Autodesk Inventor part; units mm, degrees
ref_plane "YZ Plane" through (0, 0, 0) normal (1, 0, 0) x (0, 1, 0)
ref_plane "XZ Plane" through (0, 0, 0) normal (0, 1, 0) x (-1, 0, 0)
ref_plane "XY Plane" through (0, 0, 0) normal (0, 0, 1) x (1, 0, 0)
sketch "Sketch1" plane through (0, 0, 0) normal (1, 0, 0) x (0, 1, 0)
  circle A0 centre (0, -12.7) radius 2.0955
  line L0 (0, 6.35) -> (76.2, 6.35)
  circle A1 centre (0, -38.1) radius 2.0955
  line L1 (-59.2019, -57.15) -> (76.2, -57.15)
  line L2 (76.2, 6.35) -> (96.8375, 6.35)
  line L3 (100.0125, 3.175) -> (100.0125, 1.3151)
  line L4 (95.5224, -3.175) -> (76.1708, -3.175)
  line L5 (76.1708, -47.625) -> (95.5224, -47.625)
  line L6 (100.0125, -52.1151) -> (100.0125, -53.975)
  line L7 (96.8375, -57.15) -> (76.2, -57.15)
  line L8 (99.0826, -0.9299) -> (97.7674, -2.2451)
  line L9 (97.7674, -48.5549) -> (99.0826, -49.8701)
  arc A2 (100.0125, 3.175) -> (96.8375, 6.35) centre (96.8375, 3.175) ccw
  arc A3 (99.0826, -0.9299) -> (100.0125, 1.3151) centre (96.8375, 1.3151) ccw
  arc A4 (95.5224, -3.175) -> (97.7674, -2.2451) centre (95.5224, 0) ccw
  arc A5 (97.7674, -48.5549) -> (95.5224, -47.625) centre (95.5224, -50.8) ccw
  arc A6 (100.0125, -52.1151) -> (99.0826, -49.8701) centre (96.8375, -52.1151) ccw
  arc A7 (96.8375, -57.15) -> (100.0125, -53.975) centre (96.8375, -53.975) ccw
  line L10 (59.0099, -3.175) -> (76.1708, -3.175)
  line L11 (76.1708, -47.625) -> (59.0099, -47.625)
  line L12 (0, 6.35) -> (-60.325, 6.35)
  arc A8 (-60.325, 6.35) -> (-59.8788, -6.3343) centre (-60.325, 0) ccw
  arc A9 (-59.8927, -44.5648) -> (-59.2019, -57.15) centre (-60.325, -50.9001) ccw
  line L13 (6.35, -12.7) -> (6.35, -38.1)
  line L14 (-5.5228, -38.1) -> (-5.5228, -12.0308)
  line L15 (-59.8788, -6.3343) -> (-15.0243, -3.175)
  line L16 (15.875, -3.175) -> (59.0099, -3.175)
  line L17 (15.875, -47.625) -> (59.0099, -47.625)
  line L18 (15.875, -3.175) -> (6.35, -12.7)
  line L19 (6.35, -38.1) -> (15.875, -47.625)
  line L20 (-5.5228, -38.1) -> (-15.0478, -47.625)
  line L21 (-15.0243, -3.175) -> (-5.5228, -12.0308)
  line L22 (-15.0478, -47.625) -> (-59.8927, -44.5648)
  circle A10 centre (-50.8, 0) radius 2.0955
  circle A11 centre (-50.8, -50.8) radius 2.0955
  point P0 (5.4993, -3.175)
  point P1 (0, -57.15)
  point P2 (5.4993, -47.625)
  point P3 (100.0125, -3.175)
  point P4 (100.0125, -47.625)
  point P5 (100.0125, -57.15)
  point P6 (100.0125, 0)
  point P7 (96.8375, -3.175)
  point P8 (96.8375, -47.625)
  point P9 (100.0125, -50.8)
  point P10 (38.1, 6.35)
  point P11 (-5.5228, -2.5058)
  point P12 (-5.5228, -47.625)
  point P13 (85.8466, -3.175)
  point P14 (6.35, -3.175)
  point P15 (6.35, -47.625)
  point P16 (0, 0)
  dimension "d0" = 4.191
  dimension "d6" = 4.191
  dimension "d15" = 3.175
  dimension "d16" = 3.175
  dimension "d17" = 3.175
  dimension "d18" = 3.175
  dimension "d19" = 3.175
  dimension "d29" = 9.525
  dimension "d30" = 9.525
  dimension "d31" = 9.525
  dimension "d32" = 9.525
  dimension "d34" = 9.525
  dimension "d35" = 9.525
  dimension "d36" = 9.525
  dimension "d37" = 9.525
  dimension "d38" = 9.525
  dimension "d39" = 12.7
  dimension "d40" = 12.7
  dimension "d41" = 4.191
  dimension "d42" = 4.191
  dimension "d43" = 12.7
  dimension "d44" = 0
  dimension "d45" = 25.4
extrude "Extrusion1" add sketch "Sketch1" along normal blind 1.5875
equation "\"d33\" = d31"
properties part number "Ring Guard" material "Acetal Resin, White"
Here's how the part is built. I have some questions about the finished solid (model axes, mm). A direction names the side the tool comes from. Coordinates: 2 decimals unless noted, no trailing zeros. Write each loop counter-clockwise with the first axis right and the second up, starting at its lowest first coordinate (ties: lowest second). Pieces come first, ordered by that corner, then holes.
Item 1: On a 3-axis mill with a long thin cutter (end or side, diameter ignored), from which of +Z, -Z, +X, -X, +Y, -Y can I reach the whole of each face in a straight line? I mean faces 4 (the flat face through (0.783, -37.156, -46.116)), 5 (the flat face through (0, 4, -25)), 6 (the flat face through (0.78, 11.18, -7.87)). Say none if no direction works.
Item 2: I want a section at C-C on y = 0. Write out the boundary of the cut face in (x, z).
Item 3: I want a section at B-B on x = 0.75. Count the separate pieces of the cut face and the enclosed holes in it, and give its area (3 significant figures).
Item 4: If I drill on line 1 (Z direction, x = 1.05, y = 0); line 2 (Z direction, x = 0.4, y = -60); line 3 (Z direction, x = 1.1, y = -50.8), over which ranges is the centre line in solid material (lowest first)?
Item 5: If we mould it in two halves opening along Y, with no side actions, what happens to faces 1 (the cylindrical face through (0.783, -52.893, -0.092)), 2 (the cylindrical face through (0.8, 99.1, 5.4)), 3 (the flat face through (1.588, 4, -25))? For each: +Y half, -Y half, draft (parallel to the pull), parting line (faces both ways), or undercut.
Item 6: I want a section at D-D on y = -50.8. Write out the boundary of the cut face in (x, z), and give its area (3 significant figures).
Item 7: Will these pins go through, and if not, where does the flat tip stop? pin 1 (0.8 mm diameter, centred on x = 1, y = 14.5, fed in from -Z); pin 2 (2.5 mm diameter, centred on y = -50.8, z = -50.8, fed in from -X); pin 3 (6.5 mm diameter, centred on y = 0, z = -38.1, fed in from +X); pin 4 (0.5 mm diameter, centred on x = 0.5, z = -25.5, fed in from +Y).
Findings below:
1. face 4: +X, -X
1. face 5: +Z, -Z, -X, +Y, -Y
1. face 6: +X, -X, +Y
2. outline: (0, -57.15) - (1.59, -57.15) - (1.59, -40.2) - (0, -40.2) - close; (0, -36) - (1.59, -36) - (1.59, -14.8) - (0, -14.8) - close; (0, -10.6) - (1.59, -10.6) - (1.59, 6.35) - (0, 6.35) - close
3. separate pieces: 1
3. enclosed holes: 4
3. area: 3,960 mm2
4. line 1: z = -57.15 to -40.2, -36 to -14.8, -10.6 to 6.35
4. line 2: z = -57.24 to -44.56, -6.34 to 6.35
4. line 3: z = -57.15 to -52.9, -48.7 to -45.19, -5.69 to -2.1, 2.1 to 6.35
5. face 1: undercut
5. face 2: +Y half
5. face 3: draft
6. outline: (0, -57.15) - (1.59, -57.15) - (1.59, -52.9) - (0, -52.9) - close; (0, -48.7) - (1.59, -48.7) - (1.59, -45.19) - (0, -45.19) - close; (0, -5.69) - (1.59, -5.69) - (1.59, -2.1) - (0, -2.1) - close; (0, 2.1) - (1.59, 2.1) - (1.59, 6.35) - (0, 6.35) - close
6. area: 24.8 mm2
7. pin 1: stops at z = -57.15
7. pin 2: passes through
7. pin 3: stops at x = 1.59
7. pin 4: stops at y = 6.35
